Can you work these out from the model? Positions are in its coordinate system, mm. Round coordinates to 2 decimals unless told otherwise and drop trailing zeros. Order: outer loops, then holes, each group sorted by start corner. A loop starts at its lowest first (then second) coordinate and runs counter-clockwise, first axis right, second up. Notation, with made-up numbers: M -34.75,-10 L -18.75,-10 A17 ccw -18.75,-6 Z; hole C -28,30.25 d3. An arc over 180 degrees is marked long. Answer as a JSON object with one key per item and string values. Group by question number.
```python
from build123d import *

# Parameters (mm, degrees)
F0_R     = 1.5875
F1_DEPTH = 3.048


with BuildPart() as f1:
    # F0 (on Front) → F1 (new body)
    with BuildSketch(Plane.XZ):
        with BuildLine():
            ThreePointArc((-36.0296212806, 9.5769268066), (-36.9595572504, 7.3318627763), (-39.2046212806, 6.4019268066))
            Line((-39.2046212806, 6.4019268066), (-39.2046212806, -6.2980731934))
            ThreePointArc((-39.2046212806, -6.2980731934), (-28.7097632336, -2.3341428168), (-23.4559617675, 7.57809001))
            ThreePointArc((-23.4559617675, 7.57809001), (-23.3612378861, 8.5755139973), (-23.3296212806, 9.5769268066))
            ThreePointArc((-23.3296212806, 9.5769268066), (-23.3612377133, 10.5783368816), (-23.4559610776, 11.5757581675))
            ThreePointArc((-23.4559610776, 11.5757581675), (-28.7097611781, 21.4879946188), (-39.2046212806, 25.4519268066))
            Line((-39.2046212806, 25.4519268066), (-39.2046212806, 12.7519268066))
            ThreePointArc((-39.2046212806, 12.7519268066), (-36.9595572504, 11.8219908368), (-36.0296212806, 9.5769268066))
        make_face()
        with BuildLine():
            Line((-39.2046212806, -6.2980731934), (-39.2046212806, 6.4019268066))
            ThreePointArc((-39.2046212806, 6.4019268066), (-42.3796212806, 9.5769268066), (-39.2046212806, 12.7519268066))
            Line((-39.2046212806, 12.7519268066), (-39.2046212806, 25.4519268066))
            ThreePointArc((-39.2046212806, 25.4519268066), (-49.699208832, 21.4882347585), (-54.9531899929, 11.5764788854))
            ThreePointArc((-54.9531899929, 11.5764788854), (-55.0796212766, 9.5772873178), (-54.9532807938, 7.57809001))
            ThreePointArc((-54.9532807938, 7.57809001), (-49.6994793277, -2.3341428168), (-39.2046212806, -6.2980731934))
        make_face()
        with BuildLine():
            ThreePointArc((-23.4559617675, 7.57809001), (-28.7097632336, -2.3341428168), (-39.2046212806, -6.2980731934))
            Line((-39.2046212806, -6.2980731934), (-39.2046212806, -45.0330734444))
            ThreePointArc((-39.2046212806, -45.0330734444), (-32.9184421733, -47.6368940861), (-30.3146215316, -53.9230731934))
            Line((-30.3146215316, -53.9230731934), (-2.6921212806, -53.9230731934))
            ThreePointArc((-2.6921212806, -53.9230731934), (-0.3672813563, -48.3104131178), (5.2453787194, -45.9855731934))
            Line((5.2453787194, -45.9855731934), (-20.6130872987, -45.4314633533))
            ThreePointArc((-20.6130872987, -45.4314633533), (-26.4219186802, -42.7228782392), (-28.3447482622, -36.6088221602))
            Line((-28.3447482622, -36.6088221602), (-23.4559617675, 7.57809001))
        make_face()
        with BuildLine():
            Line((-39.2046212806, -45.0330734444), (-39.2046212806, -6.2980731934))
            ThreePointArc((-39.2046212806, -6.2980731934), (-49.6994793277, -2.3341428168), (-54.9532807938, 7.57809001))
            Line((-54.9532807938, 7.57809001), (-48.0407045344, -54.9006867526))
            ThreePointArc((-48.0407045344, -54.9006867526), (-45.8274258163, -47.9925963474), (-39.2046212806, -45.0330734444))
        make_face()
        with BuildLine():
            Line((-39.2046212806, 50.8519268066), (-39.2046212806, 25.4519268066))
            ThreePointArc((-39.2046212806, 25.4519268066), (-28.7097611781, 21.4879946188), (-23.4559610776, 11.5757581675))
            Line((-23.4559610776, 11.5757581675), (-29.6832617971, 60.6402490134))
            ThreePointArc((-29.6832617971, 60.6402490134), (-29.6805314532, 60.5086004922), (-29.6796212806, 60.3769268066))
            ThreePointArc((-29.6796212806, 60.3769268066), (-32.4694291898, 53.6417347158), (-39.2046212806, 50.8519268066))
        make_face()
        with BuildLine():
            ThreePointArc((-54.9531899929, 11.5764788854), (-49.699208832, 21.4882347585), (-39.2046212806, 25.4519268066))
            Line((-39.2046212806, 25.4519268066), (-39.2046212806, 50.8519268066))
            ThreePointArc((-39.2046212806, 50.8519268066), (-46.0243552101, 53.7273513216), (-48.7265815015, 60.6175479864))
            Line((-48.7265815015, 60.6175479864), (-54.9531899929, 11.5764788854))
        make_face()
        with Locations((-43.2879850268, 46.1021268066)):
            Circle(F0_R, mode=Mode.SUBTRACT)
        with BuildLine():
            Line((-39.2046212806, -50.7480731934), (-39.2046212806, -45.0330734444))
            ThreePointArc((-39.2046212806, -45.0330734444), (-45.8274258163, -47.9925963474), (-48.0407045344, -54.9006867526))
            ThreePointArc((-48.0407045344, -54.9006867526), (-45.1350981267, -60.5458777291), (-39.2046212806, -62.8130729425))
            Line((-39.2046212806, -62.8130729425), (-38.8245213576, -62.8049434687))
            ThreePointArc((-38.8245213576, -62.8049434687), (-32.7854630898, -60.0733986856), (-30.3146215316, -53.9230731934))
            Line((-30.3146215316, -53.9230731934), (-36.0296212806, -53.9230731934))
            ThreePointArc((-36.0296212806, -53.9230731934), (-41.4496853109, -56.1681372237), (-39.2046212806, -50.7480731934))
        make_face()
        with BuildLine():
            ThreePointArc((-48.7265815015, 60.6175479864), (-46.0243552101, 53.7273513216), (-39.2046212806, 50.8519268066))
            ThreePointArc((-39.2046212806, 50.8519268066), (-32.4694291898, 53.6417347158), (-29.6796212806, 60.3769268066))
            ThreePointArc((-29.6796212806, 60.3769268066), (-29.6805314532, 60.5086004922), (-29.6832617971, 60.6402490134))
            ThreePointArc((-29.6832617971, 60.6402490134), (-39.2159757678, 69.9019200389), (-48.7265815015, 60.6175479864))
        make_face()
        with BuildLine():
            ThreePointArc((-36.0296212806, 60.3769268066), (-36.9595572504, 58.1318627763), (-39.2046212806, 57.2019268066))
            ThreePointArc((-39.2046212806, 57.2019268066), (-41.4496853109, 62.6219908368), (-36.0296212806, 60.3769268066))
        make_face(mode=Mode.SUBTRACT)
        with BuildLine():
            Line((-2.6921212806, -53.9230731934), (-30.3146215316, -53.9230731934))
            ThreePointArc((-30.3146215316, -53.9230731934), (-32.7854630898, -60.0733986856), (-38.8245213576, -62.8049434687))
            Line((-38.8245213576, -62.8049434687), (5.4151049958, -61.8587583712))
            ThreePointArc((5.4151049958, -61.8587583712), (-0.3069497981, -59.5954231725), (-2.6921212806, -53.9230731934))
        make_face()
        with BuildLine():
            ThreePointArc((5.2453787194, -45.9855731934), (-0.3672813563, -48.3104131178), (-2.6921212806, -53.9230731934))
            ThreePointArc((-2.6921212806, -53.9230731934), (-0.3069497981, -59.5954231725), (5.4151049958, -61.8587583712))
            ThreePointArc((5.4151049958, -61.8587583712), (10.9177286984, -59.4754017108), (13.1828787194, -53.9230731934))
            ThreePointArc((13.1828787194, -53.9230731934), (10.858038795, -48.3104131178), (5.2453787194, -45.9855731934))
        make_face()
        with BuildLine():
            ThreePointArc((8.4203787194, -53.9230731934), (5.2453787194, -57.0980731934), (2.0703787194, -53.9230731934))
            ThreePointArc((2.0703787194, -53.9230731934), (5.2453787194, -50.7480731934), (8.4203787194, -53.9230731934))
        make_face(mode=Mode.SUBTRACT)
        with BuildLine():
            ThreePointArc((-39.2046212806, -62.8130729425), (-39.0145278564, -62.8110403417), (-38.8245213576, -62.8049434687))
            Line((-38.8245213576, -62.8049434687), (-39.2046212806, -62.8130729425))
        make_face()
        with BuildLine():
            ThreePointArc((-30.3146215316, -53.9230731934), (-32.9184421733, -47.6368940861), (-39.2046212806, -45.0330734444))
            Line((-39.2046212806, -45.0330734444), (-39.2046212806, -50.7480731934))
            ThreePointArc((-39.2046212806, -50.7480731934), (-36.9595572504, -51.6780091632), (-36.0296212806, -53.9230731934))
            Line((-36.0296212806, -53.9230731934), (-30.3146215316, -53.9230731934))
        make_face()
    extrude(amount=F1_DEPTH)


solid = f1.part
```
1) We'd pull the mould along X, two halves only. Please class faces 1 (the face through (-25.935, -1.503, -14.825)), 2 (the face through (-55.08, -1.5, 9.61)), 3 (the face through (-41.774, -1.503, 46.579)), 4 (the face through (-39, -1.5, 69.9)): +X half, -X half, draft (parallel to the pull), parting line (faces both ways), or undercut.
2) If we section it at B-B on y = -0.6: Count the separate pieces of the cut face and the enclosed holes in it, plus the area to 3 significant figures.
3) If we section it at A-A on x = -27: Write out the boundary of the cut face in (y, z).
4) I need wall thicknesses on line 1 along X through (y, z) = (-2.15, -53); line 2 along Z through (x, y) = (4, -0.9); line 3 along Z through (x, y) = (3.5, -1.1). Which ranges of each line are inside material? Lowest first, please.
5) If we section it at C-C on z = 59: Write out the boundary of the cut face in (x, y).
6) For pin 1 (1.5 mm diameter, centred on x = 5.5, y = -2, fed in from -Z), with a flat end and sliding along its axis, tell me the tip position at first contact or that it passes through.
7) If we section it at D-D on x = -17: Write out the boundary of the cut face in (y, z), plus the area to 3 significant figures.
Findings:
{
 "1": {"face 1": "+X half", "face 2": "-X half", "face 3": "undercut", "face 4": "parting line"},
 "2": {"separate pieces": "1", "enclosed holes": "5", "area": "3,730 mm^2"},
 "3": {"outline": "M -3.05,-62.55 L 0,-62.55 L 0,-41.98 L -3.05,-41.98 Z; M -3.05,-24.45 L 0,-24.45 L 0,39.5 L -3.05,39.5 Z"},
 "4": {"line 1": "x = -48.25 to -42.24, -36.17 to 2.21, 8.28 to 13.13", "line 2": "z = -61.89 to -56.84, -51 to -45.96", "line 3": "z = -61.9 to -56.58, -51.27 to -45.95"},
 "5": {"outline": "M -48.93,-3.05 L -42.07,-3.05 L -42.07,0 L -48.93,0 Z; M -36.34,-3.05 L -29.48,-3.05 L -29.48,0 L -36.34,0 Z"},
 "6": {"pin 1": "stops at z = -61.87"},
 "7": {"outline": "M -3.05,-62.34 L 0,-62.34 L 0,-45.51 L -3.05,-45.51 Z", "area": "51.3 mm^2"}
}
